Build history of the part. All positions in model axes, mm. Round coordinates to 2 decimals unless told otherwise and drop trailing zeros. Write each loop counter-clockwise with the first axis right and the second up, starting at its lowest first coordinate (ties: lowest second). Pieces come first, ordered by that corner, then holes.
Item 1: Band-saw the part on A-A, the plane y = -60. Write the cut outline in (x, z), then the cut area to 3 significant figures.
Item 2: Band-saw the part on B-B, the plane x = 37.5. Write the cut outline in (y, z), then the cut area to 3 significant figures.
Item 3: Band-saw the part on C-C, the plane x = -57.5. Write the cut outline in (y, z), then the cut area to 3 significant figures.
Item 4: Wall check: probe 1 along Y at (x, z) = (-57.5, 7); probe 2 along Y at (x, z) = (37.5, 4.75). Give the ranges that are in metal, low to high.
```python
from build123d import *

# Parameters (mm, degrees)
SKETCH1_W              = 130
SKETCH1_H              = 150
EXTRUDE1_DEPTH         = 16
M6_TAPPED_HOLE1_D      = 5
M5_TAPPED_HOLE1_D      = 4.2
M5_TAPPED_HOLE1_DEPTH  = 16
M10_TAPPED_HOLE1_D     = 8.5
M10_TAPPED_HOLE1_DEPTH = 27.5
M10_TAPPED_HOLE1_TIP   = 2.553657631
M10_TAPPED_HOLE2_D     = 8.5
M10_TAPPED_HOLE2_DEPTH = 27.5
M10_TAPPED_HOLE2_TIP   = 2.553657631


with BuildPart() as part:
    # Sketch1 → Extrude1 (new body)
    with BuildSketch(Plane.XY):
        Rectangle(SKETCH1_W, SKETCH1_H)
    extrude(amount=EXTRUDE1_DEPTH)

    # M6 Tapped Hole1 (through all)
    with Locations(Plane.XY.offset(16)):
        with Locations((-57.5, 60), (-57.5, 0), (-57.5, -60), (57.5, -60), (57.5, 0), (57.5, 60)):
            Hole(M6_TAPPED_HOLE1_D / 2)

    # M5 Tapped Hole1
    with Locations(Plane.XY.offset(16)):
        with Locations((-37.5, 50), (37.5, 50), (37.5, -50), (-37.5, -50)):
            Hole(M5_TAPPED_HOLE1_D / 2, depth=M5_TAPPED_HOLE1_DEPTH)

    # M10 Tapped Hole1
    with Locations(Plane(origin=(0, 0, 0), x_dir=(-1, 0, 0), z_dir=(0, 0, -1))):
        with Locations((-15, 25)):
            Hole(M10_TAPPED_HOLE1_D / 2, depth=M10_TAPPED_HOLE1_DEPTH)
            with Locations((0, 0, -(M10_TAPPED_HOLE1_DEPTH + M10_TAPPED_HOLE1_TIP / 2))):  # 118° drill point
                Cone(0, M10_TAPPED_HOLE1_D / 2, M10_TAPPED_HOLE1_TIP, mode=Mode.SUBTRACT)

    # M10 Tapped Hole2
    with Locations(Plane(origin=(0, 0, 0), x_dir=(-1, 0, 0), z_dir=(0, 0, -1))):
        with Locations((15, 25)):
            Hole(M10_TAPPED_HOLE2_D / 2, depth=M10_TAPPED_HOLE2_DEPTH)
            with Locations((0, 0, -(M10_TAPPED_HOLE2_DEPTH + M10_TAPPED_HOLE2_TIP / 2))):  # 118° drill point
                Cone(0, M10_TAPPED_HOLE2_D / 2, M10_TAPPED_HOLE2_TIP, mode=Mode.SUBTRACT)


solid = part.part
```
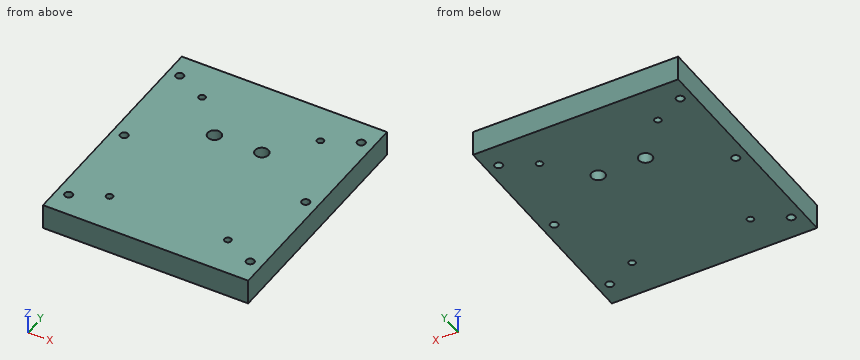
Results:
1. outline: (-65, 0) - (-60, 0) - (-60, 16) - (-65, 16) - close; (-55, 0) - (55, 0) - (55, 16) - (-55, 16) - close; (60, 0) - (65, 0) - (65, 16) - (60, 16) - close
1. area: 1,920 mm2
2. outline: (-75, 0) - (-52.1, 0) - (-52.1, 16) - (-75, 16) - close; (-47.9, 0) - (47.9, 0) - (47.9, 16) - (-47.9, 16) - close; (52.1, 0) - (75, 0) - (75, 16) - (52.1, 16) - close
2. area: 2,270 mm2
3. outline: (-75, 0) - (-62.5, 0) - (-62.5, 16) - (-75, 16) - close; (-57.5, 0) - (-2.5, 0) - (-2.5, 16) - (-57.5, 16) - close; (2.5, 0) - (57.5, 0) - (57.5, 16) - (2.5, 16) - close; (62.5, 0) - (75, 0) - (75, 16) - (62.5, 16) - close
3. area: 2,160 mm2
4. probe 1: y = -75 to -62.5, -57.5 to -2.5, 2.5 to 57.5, 62.5 to 75
4. probe 2: y = -75 to -52.1, -47.9 to 47.9, 52.1 to 75
